The figure shows three views and two pictorial views of one solid part (mm, origin at its lowest corner). Answer the questions. A direction names the side the tool comes from. Round coordinates to 2 decimals unless told otherwise and drop trailing zeros. Order: outer loops, then holes, each group sorted by start corner. A loop starts at its lowest first (then second) coordinate and runs counter-clockwise, first axis right, second up. Notation, with made-up numbers: (51.25, 39.25) -> (56.25, 39.25) arc R25 ccw to (56.25, 69.25) -> close; hole circle Ø8 at (74.25, -6.75). An arc over 180 degrees is marked (long way). Answer as a JSON object with one key per item and string values. Group by question number.
Item 1: Section A-A, the plane x = 30.5 is taken. Write down the section's boundary in (y, z).
Item 2: Section B-B, the plane z = 17.5 is taken. Write down the section's boundary in (x, y).
Item 3: Section C-C, the plane y = 2.75 is taken. Write down the section's boundary in (x, z), plus the area to 3 significant figures.
Item 4: Section D-D, the plane x = 11 is taken. Write down the section's boundary in (y, z), plus the area to 3 significant figures.
Item 5: Given P1, Ø10, axis at x = 15, z = 10.5, coming from the +Y side; P2, Ø4, axis at x = 28, y = 9, coming from the +Z side; P3, Ø4.5, axis at y = 2, z = 11.5, coming from the -X side, each flat-ended and moving along its own axis, determine where each tip first touches the part or whether it passes through.
Item 6: For the marked faces 1 and 2, determine the directions among +Z, -Z, +X, -X, +Y, -Y from which every point of the face is accessible in a straight line to the end or side of a thin tool.
Item 7: Consider probe 1 along Z at (x, y) = (34, 1.5); probe 2 along Y at (x, z) = (31.5, 6.5); probe 3 along Z at (x, y) = (17.5, 5). Determine where each line is inside the solid, lowest interval first. Write a range as from..to.
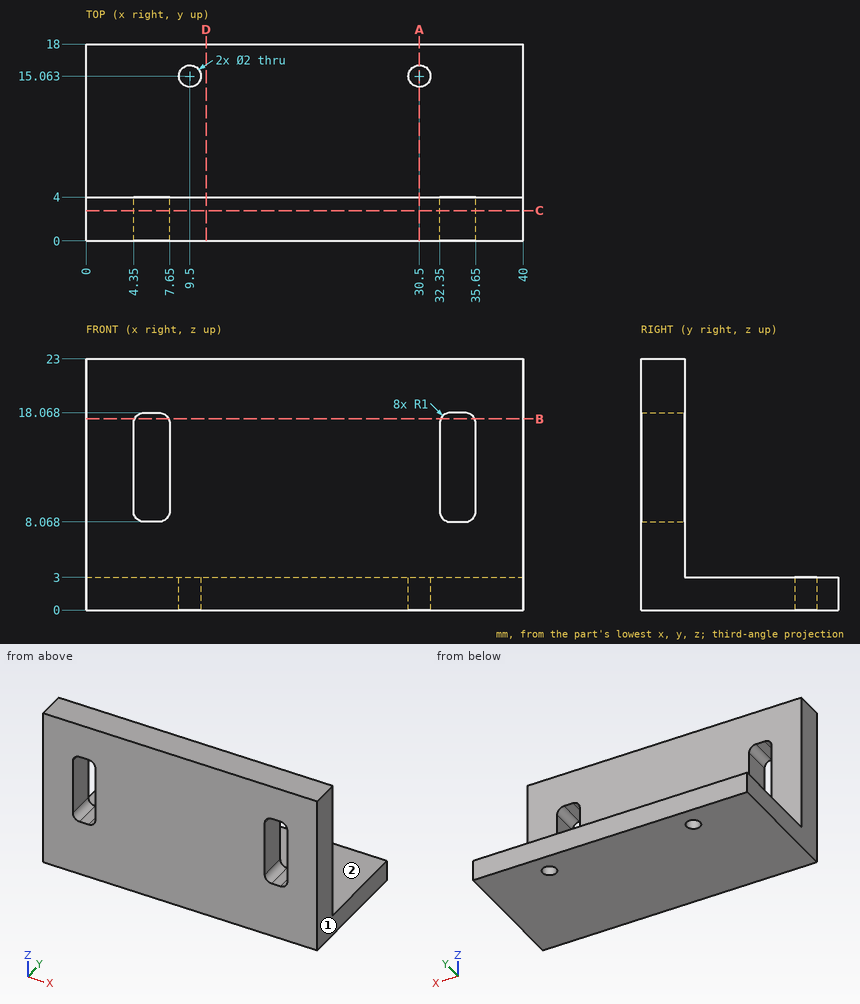
Values found:
{
 "1": {"outline": "(0, 0) -> (14.06, 0) -> (14.06, 3) -> (4, 3) -> (4, 23) -> (0, 23) -> close; (16.06, 0) -> (18, 0) -> (18, 3) -> (16.06, 3) -> close"},
 "2": {"outline": "(0, 0) -> (4.45, 0) -> (4.45, 4) -> (0, 4) -> close; (7.55, 0) -> (32.45, 0) -> (32.45, 4) -> (7.55, 4) -> close; (35.55, 0) -> (40, 0) -> (40, 4) -> (35.55, 4) -> close"},
 "3": {"outline": "(0, 0) -> (40, 0) -> (40, 23) -> (0, 23) -> close; hole (4.35, 9.07) arc R1 ccw to (5.35, 8.07) -> (6.65, 8.07) arc R1 ccw to (7.65, 9.07) -> (7.65, 17.07) arc R1 ccw to (6.65, 18.07) -> (5.35, 18.07) arc R1 ccw to (4.35, 17.07) -> close; hole (32.35, 9.07) arc R1 ccw to (33.35, 8.07) -> (34.65, 8.07) arc R1 ccw to (35.65, 9.07) -> (35.65, 17.07) arc R1 ccw to (34.65, 18.07) -> (33.35, 18.07) arc R1 ccw to (32.35, 17.07) -> close", "area": "856 mm2"},
 "4": {"outline": "(0, 0) -> (18, 0) -> (18, 3) -> (4, 3) -> (4, 23) -> (0, 23) -> close", "area": "134 mm2"},
 "5": {"P1": "y = 4", "P2": "z = 3", "P3": "x = 0"},
 "6": {"face 1": "+Z, -Z, +X, +Y, -Y", "face 2": "+Z, +X, -X, +Y"},
 "7": {"probe 1": "0..8.07, 18.07..23", "probe 2": "0..4", "probe 3": "0..3"}
}
